```python
from build123d import *

# Parameters (mm, degrees)
SKIZZE1_R                       = 1
AUFSATZ_LINEAR_AUSTRAGEN1_DEPTH = 4
SCHNITT_LINEAR_AUSTRAGEN1_DEPTH = 6
SCHNITT_LINEAR_AUSTRAGEN2_DEPTH = 3


with BuildPart() as part:
    # Skizze1 → Aufsatz-Linear austragen1 (new body)
    with BuildSketch(Plane.XY):
        with BuildLine():
            ThreePointArc((-73.08156136, 10.209205546), (-85.925298124, 0), (-73.08156136, -10.209205546))
            ThreePointArc((-73.08156136, -10.209205546), (-37.708269243, -6.148967962), (-2.327018144, -10.139255556))
            ThreePointArc((-2.327018144, -10.139255556), (10.402860985, 0), (-2.327018144, 10.139255556))
            ThreePointArc((-2.327018144, 10.139255556), (-37.708269243, 6.148967962), (-73.08156136, 10.209205546))
        make_face()
        Circle(SKIZZE1_R, mode=Mode.SUBTRACT)
    extrude(amount=AUFSATZ_LINEAR_AUSTRAGEN1_DEPTH)

    # Skizze2 → Schnitt-Linear austragen1 (cut)
    with BuildSketch(Plane.XY.offset(4)):
        with BuildLine():
            ThreePointArc((-1.655947518, 7.215274671), (-7.402860985, 0), (-1.655947518, -7.215274671))
            ThreePointArc((-1.655947518, -7.215274671), (-37.711235128, -3.148969428), (-73.758412133, -7.286557255))
            ThreePointArc((-73.758412133, -7.286557255), (-82.925298124, 0), (-73.758412133, 7.286557255))
            ThreePointArc((-73.758412133, 7.286557255), (-37.711235128, 3.148969428), (-1.655947518, 7.215274671))
        make_face()
    extrude(amount=-SCHNITT_LINEAR_AUSTRAGEN1_DEPTH, mode=Mode.SUBTRACT)

    # Skizze6 → Schnitt-Linear austragen2 (cut)
    with BuildSketch(Plane.XY.offset(4)):
        Polygon((1.165582934, 1.788027089), (1.018080563, 2.19148446), (0.614623192, 2.043982089), (0.359428626, 2.389540381), (0.013870334, 2.134345816), (-0.32834208, 2.394009952), (-0.588006216, 2.051797538), (-0.989512463, 2.204531074), (-1.142245999, 1.803024827), (-1.570518432, 1.836454199), (-1.603947805, 1.408181766), (-2.024290337, 1.319598727), (-1.935707298, 0.899256194), (-2.314066279, 0.695837214), (-2.110647298, 0.317478234), (-2.416370332, 0.015703108), (-2.114595207, -0.290019926), (-2.322914432, -0.66570317), (-1.947231188, -0.874022395), (-2.04126982, -1.293178136), (-1.622114079, -1.387216768), (-1.594253667, -1.815887501), (-1.165582934, -1.788027089), (-1.018080563, -2.19148446), (-0.614623192, -2.043982089), (-0.359428626, -2.389540381), (-0.013870334, -2.134345816), (0.32834208, -2.394009952), (0.588006216, -2.051797538), (0.989512463, -2.204531074), (1.142245999, -1.803024827), (1.570518432, -1.836454199), (1.603947805, -1.408181766), (2.024290337, -1.319598727), (1.935707298, -0.899256194), (2.314066279, -0.695837214), (2.110647298, -0.317478234), (2.416370332, -0.015703108), (2.114595207, 0.290019926), (2.322914432, 0.66570317), (1.947231188, 0.874022395), (2.04126982, 1.293178136), (1.622114079, 1.387216768), (1.594253667, 1.815887501), align=None)
    extrude(amount=-SCHNITT_LINEAR_AUSTRAGEN2_DEPTH, mode=Mode.SUBTRACT)


solid = part.part
```
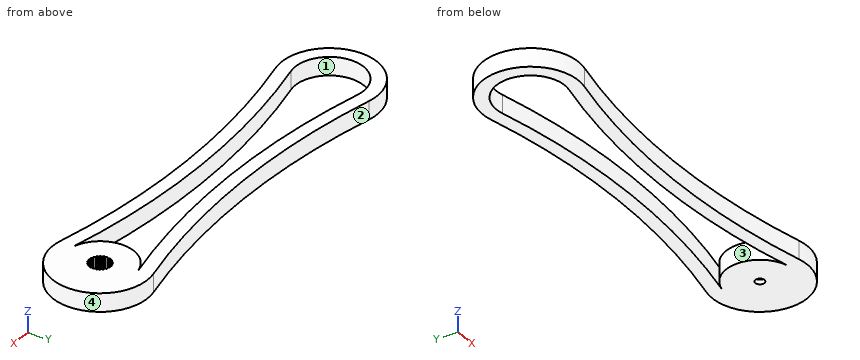
Build history of the part. All positions in model axes, mm. Face numbers are marked on the shaded views. Round coordinates to 2 decimals unless told otherwise and drop trailing zeros. Order: outer loops, then holes, each group sorted by start corner. A loop starts at its lowest first (then second) coordinate and runs counter-clockwise, first axis right, second up. Notation, with made-up numbers: (55, 11.25) -> (72, 11.25) arc R21 ccw to (72, 18.25) -> close; hole circle Ø6 at (15, 15). An arc over 180 degrees is marked (long way). Answer in a Markdown table with one row per item.
1) Band-saw the part on B-B on x = -43. Give the cut face in (y, z), and give its area (3 significant figures).
Values:
| item | result |
|---|---|
| outline | (-6.24, 0) -> (-3.24, 0) -> (-3.24, 4) -> (-6.24, 4) -> close; (3.24, 0) -> (6.24, 0) -> (6.24, 4) -> (3.24, 4) -> close |
| area | 24.0 mm2 |
2) Band-saw the part on D-D on z = 1.8. Give the number of separate pieces and of enclosed holes in the cut face, and give its area (3 significant figures).
Values:
| item | result |
|---|---|
| separate pieces | 1 |
| enclosed holes | 2 |
| area | 781 mm2 |
3) Mould opens along Y. For the marked faces 1, 2, 3 and 4 say: released by +Y, released by -Y, zero draft, split by the parting line, or undercut.
Values:
| item | result |
|---|---|
| face 1 | undercut |
| face 2 | released by +Y |
| face 3 | undercut |
| face 4 | split by the parting line |
4) Pin check, flat tips, straight feed: P1, Ø1, axis at y = 6, z = 2.5, coming from the +X side; P2, Ø1, axis at x = -67.5, z = 1, coming from the +Y side; P3, Ø1.4, axis at x = -0.5, y = -1, coming from the +Z side. Stop position of each tip, or through.
Values:
| item | result |
|---|---|
| P1 | x = 8.83 |
| P2 | y = 9.12 |
| P3 | z = 1 |
5) Wall check: L1, parallel to Y at x = 0, z = 0.65; L2, parallel to Y at x = -39.5, z = 0.7; L3, parallel to X at y = -0.25, z = 0.2. Give the ranges that are in metal, low to high.
Values:
| item | result |
|---|---|
| L1 | -10.4 to -1, 1 to 10.4 |
| L2 | -6.16 to -3.16, 3.16 to 6.16 |
| L3 | -85.92 to -82.92, -7.4 to -0.97, 0.97 to 10.4 |
6) Band-saw the part on A-A on y = 8.75. Give the cut face in (x, z).
Values:
| item | result |
|---|---|
| outline | (-81.21, 0) -> (-66.06, 0) -> (-66.06, 4) -> (-81.21, 4) -> close; (-9.05, 0) -> (5.63, 0) -> (5.63, 4) -> (-9.05, 4) -> close |
